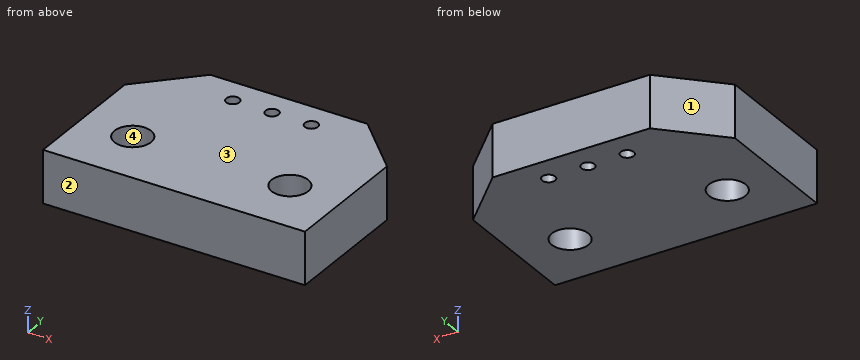
```python
from build123d import *

# Parameters (mm, degrees)
BOSS_EXTRUDE1_DEPTH            = 2
F_1_4_1_4_DIAMETER_HOLE1_D     = 1.4
F_1_4_1_4_DIAMETER_HOLE1_DEPTH = 10
F_1_4_1_4_DIAMETER_HOLE1_TIP   = 0.420602433
F_0_5_0_5_DIAMETER_HOLE1_D     = 0.5
F_0_5_0_5_DIAMETER_HOLE1_DEPTH = 10
F_0_5_0_5_DIAMETER_HOLE1_TIP   = 0.150215155


with BuildPart() as part:
    # Sketch1 → Boss-Extrude1 (new body)
    with BuildSketch(Plane.XY):
        Polygon((1.097109919, 0), (1.097109919, 5), (3.097109919, 7), (9.097109919, 7), (11.097109919, 5), (11.097109919, 0), align=None)
    extrude(amount=BOSS_EXTRUDE1_DEPTH)

    # Ø1.4 (1.4) Diameter Hole1
    with Locations(Plane.XY.offset(2)):
        with Locations((3.097109919, 2.27502281), (9.097109919, 2.27502281)):
            Hole(F_1_4_1_4_DIAMETER_HOLE1_D / 2, depth=F_1_4_1_4_DIAMETER_HOLE1_DEPTH)
            with Locations((0, 0, -(F_1_4_1_4_DIAMETER_HOLE1_DEPTH + F_1_4_1_4_DIAMETER_HOLE1_TIP / 2))):  # 118° drill point
                Cone(0, F_1_4_1_4_DIAMETER_HOLE1_D / 2, F_1_4_1_4_DIAMETER_HOLE1_TIP, mode=Mode.SUBTRACT)

    # Ø0.5 (0.5) Diameter Hole1
    with Locations(Plane.XY.offset(2)):
        with Locations((6.097109919, 5.979300112), (4.597109919, 5.979300112), (7.597109919, 5.979300112)):
            Hole(F_0_5_0_5_DIAMETER_HOLE1_D / 2, depth=F_0_5_0_5_DIAMETER_HOLE1_DEPTH)
            with Locations((0, 0, -(F_0_5_0_5_DIAMETER_HOLE1_DEPTH + F_0_5_0_5_DIAMETER_HOLE1_TIP / 2))):  # 118° drill point
                Cone(0, F_0_5_0_5_DIAMETER_HOLE1_D / 2, F_0_5_0_5_DIAMETER_HOLE1_TIP, mode=Mode.SUBTRACT)


solid = part.part
```
Source: CAD feature listing. Evaluate the final solid. Frame: model axes, mm. Face numbers are marked on the shaded views. Round coordinates to 2 decimals unless told otherwise and drop trailing zeros. Loops run counter-clockwise (first coordinate to the right, second up) from the corner with the lowest first, then second, coordinate; pieces in that order, holes last. Notation, with made-up numbers: M 23.5,10.25 L 58.5,10.25 A8 ccw 58.5,25.25 Z; hole C 27.5,45.5 d5. An arc over 180 degrees is marked long. Use a Markdown table: item, result. Add a question column.
1. Cut plane D-D, the plane y = 5.25. Output: boundary loops of the cut face in (x, z), and give its area (3 significant figures).
2. Cut plane C-C, the plane z = 0.9. Output: boundary loops of the cut face in (x, y).
3. Cut plane B-B, the plane y = 2.75. Output: boundary loops of the cut face in (x, z).
4. Ray query, line 1 along Y through (x, z) = (3.5, 0.85); line 2 along X through (y, z) = (2.75, 1.9); line 3 along Y through (x, z) = (10.25, 1.1). Return the intervals inside material, ascending. Write a range as [from, to].
5. Cut plane A-A, the plane x = 9.5. Output: boundary loops of the cut face in (y, z).
6. Pull-direction query (Y, two-part tool) for the marked faces 1, 2, 3 and 4; classes: +Y half, -Y half, draft (parallel to the pull), parting line (faces both ways), or undercut.
7. Contact query for flat-ended pins moving along their axis: pin 1 (1.6 mm diameter, centred on x = 9.1, y = 2.28, fed in from -Z); pin 2 (1.1 mm diameter, centred on x = 3.1, y = 2.28, fed in from -Z). Output: stop coordinate, or through.
Solution:
| question | item | result |
|---|---|---|
| 1 | outline | M 1.35,0 L 10.85,0 L 10.85,2 L 1.35,2 Z |
| 1 | area | 19.0 mm2 |
| 2 | outline | M 1.1,0 L 11.1,0 L 11.1,5 L 9.1,7 L 3.1,7 L 1.1,5 Z; hole C 3.1,2.28 d1.4; hole C 4.6,5.98 d0.5; hole C 6.1,5.98 d0.5; hole C 7.6,5.98 d0.5; hole C 9.1,2.28 d1.4 |
| 3 | outline | M 1.1,0 L 2.58,0 L 2.58,2 L 1.1,2 Z; M 3.61,0 L 8.58,0 L 8.58,2 L 3.61,2 Z; M 9.61,0 L 11.1,0 L 11.1,2 L 9.61,2 Z |
| 4 | line 1 | y = [0, 1.7], [2.85, 7] |
| 4 | line 2 | x = [1.1, 2.58], [3.61, 8.58], [9.61, 11.1] |
| 4 | line 3 | y = [0, 5.85] |
| 5 | outline | M 0,0 L 1.7,0 L 1.7,2 L 0,2 Z; M 2.85,0 L 6.6,0 L 6.6,2 L 2.85,2 Z |
| 6 | face 1 | +Y half |
| 6 | face 2 | -Y half |
| 6 | face 3 | draft |
| 6 | face 4 | undercut |
| 7 | pin 1 | stops at z = 0 |
| 7 | pin 2 | passes through |
